Geometry check sheet. Reference: the model listing, model coordinates, mm. Face numbers are marked on the shaded views. Round coordinates to 2 decimals unless told otherwise and drop trailing zeros. Loops run counter-clockwise (first coordinate to the right, second up) from the corner with the lowest first, then second, coordinate; pieces in that order, holes last. Notation, with made-up numbers: (33.25, 70) -> (41.25, 70) arc R5 ccw to (41.25, 75) -> close; hole circle Ø10 at (69, 40). An arc over 180 degrees is marked (long way). Use a Markdown table: item, result. Add a question column.
Q1. Material ranges on L1, parallel to X at y = 41, z = 0; L2, parallel to X at y = 7, z = 0; L3, parallel to Y at x = -36.4, z = 0, recorded low to high.
Q2. Sectioned sample at C-C, the plane y = 36.5. Enter the section's corners in (x, z) (3 decimals), then the cut area to 3 significant figures.
Q3. Release check for a two-part mould opening along Z. For the marked faces 1, 2 and 3 record: released by +Z, released by -Z, zero draft, split by the parting line, or undercut.
Q4. Gauge pin test, flat ends, axial feed: P1, Ø12, axis at x = 10.5, z = -10, coming from the -Y side; P2, Ø6, axis at x = 21.5, z = 23.5, coming from the +Y side; P3, Ø8, axis at x = 9.5, z = -27.5, coming from the +Y side; P4, Ø24, axis at y = 20, z = 0, coming from the -X side. Record the tip position at first contact, or that the pin passes through.
Q5. Sectioned sample at B-B, the plane z = 0. Enter the section's corners in (x, y).
Q6. Sectioned sample at A-A, the plane x = 0. Enter the section's corners in (y, z), then the cut area to 3 significant figures.
Q7. Sectioned sample at D-D, the plane y = 20. Enter the section's corners in (x, z) (3 decimals), then the cut area to 3 significant figures.
```python
from build123d import *

# Parameters (mm, degrees)
SKETCH1_R           = 35.75
SKETCH1_R_2         = 34.75
BOSS_EXTRUDE1_DEPTH = 10
SKETCH2_R           = 36.8
SKETCH2_R_2         = 34.75
BOSS_EXTRUDE3_DEPTH = 2
SKETCH3_R           = 36.8
SKETCH3_R_2         = 35.8
BOSS_EXTRUDE4_DEPTH = 70
SKETCH4_W           = 1
SKETCH4_H           = 68.749981818
BOSS_EXTRUDE5_DEPTH = 50
SKETCH5_R           = 7.5
CUT_EXTRUDE1_DEPTH  = 10


with BuildPart() as part:
    # Sketch1 → Boss-Extrude1 (new body)
    with BuildSketch(Plane(origin=(0, 0, 0), x_dir=(1, 0, 0), z_dir=(0, 1, 0))):
        with Locations(Location((0, 0, 0), (0, 0, 270))):
            Circle(SKETCH1_R)
        with Locations(Location((0, 0, 0), (0, 0, 270))):
            Circle(SKETCH1_R_2, mode=Mode.SUBTRACT)
    extrude(amount=BOSS_EXTRUDE1_DEPTH)

    # Sketch2 → Boss-Extrude3 (add)
    with BuildSketch(Plane(origin=(0, 10, 0), x_dir=(1, 0, 0), z_dir=(0, 1, 0))):
        with Locations(Location((0, 0, 0), (0, 0, 270))):
            Circle(SKETCH2_R)
        with Locations(Location((0, 0, 0), (0, 0, 270))):
            Circle(SKETCH2_R_2, mode=Mode.SUBTRACT)
    extrude(amount=BOSS_EXTRUDE3_DEPTH)

    # Sketch3 → Boss-Extrude4 (add)
    with BuildSketch(Plane(origin=(0, 12, 0), x_dir=(1, 0, 0), z_dir=(0, 1, 0))):
        with Locations(Location((0, 0, 0), (0, 0, 270))):
            Circle(SKETCH3_R)
        with Locations(Location((0, 0, 0), (0, 0, 270))):
            Circle(SKETCH3_R_2, mode=Mode.SUBTRACT)
    extrude(amount=BOSS_EXTRUDE4_DEPTH)

    # Sketch4 → Boss-Extrude5 (add)
    with BuildSketch(Plane(origin=(0, 12, 0), x_dir=(1, 0, 0), z_dir=(0, 1, 0))):
        with Locations((10.5, 0)):
            Rectangle(SKETCH4_W, SKETCH4_H)
    extrude(amount=BOSS_EXTRUDE5_DEPTH)

    # Sketch5 → Cut-Extrude1 (cut)
    with BuildSketch(Plane.ZY.offset(36.8)):
        with Locations((0, 20)):
            Circle(SKETCH5_R)
    extrude(amount=-CUT_EXTRUDE1_DEPTH, mode=Mode.SUBTRACT)


solid = part.part
```
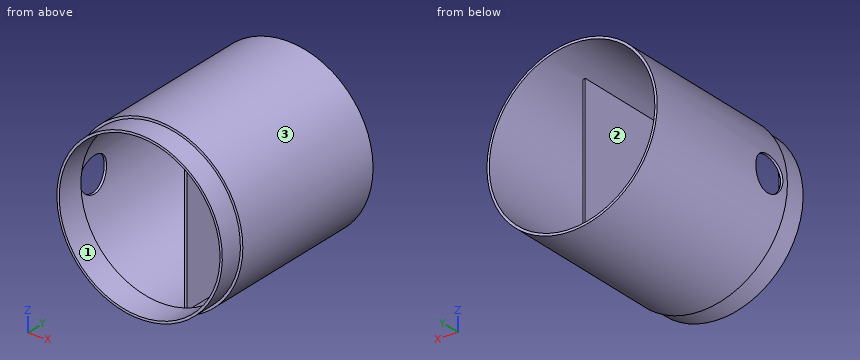
Values:
| question | item | result |
|---|---|---|
| 1 | L1 | -36.8 to -35.8, 10 to 11, 35.8 to 36.8 |
| 1 | L2 | -35.75 to -34.75, 34.75 to 35.75 |
| 1 | L3 | 10 to 12.5, 27.5 to 82 |
| 2 | outline | circle Ø73.6 at (0, 0); hole (10, -34.375) -> (10, 34.375) arc R35.8 ccw (long way) to start; hole (11, -34.068) arc R35.8 ccw to (11, 34.068) -> close |
| 2 | area | 297 mm^2 |
| 3 | face 1 | undercut |
| 3 | face 2 | undercut |
| 3 | face 3 | split by the parting line |
| 4 | P1 | y = 12 |
| 4 | P2 | y = 12 |
| 4 | P3 | y = 62 |
| 4 | P4 | x = -36.8 |
| 5 | outline | (-36.8, 10) -> (-35.75, 10) -> (-35.75, 0) -> (-34.75, 0) -> (-34.75, 12) -> (-35.8, 12) -> (-35.8, 12.5) -> (-36.8, 12.5) -> close; (-36.8, 27.5) -> (-35.8, 27.5) -> (-35.8, 82) -> (-36.8, 82) -> close; (10, 12) -> (11, 12) -> (11, 62) -> (10, 62) -> close; (34.75, 0) -> (35.75, 0) -> (35.75, 10) -> (36.8, 10) -> (36.8, 82) -> (35.8, 82) -> (35.8, 12) -> (34.75, 12) -> close |
| 6 | outline | (0, -35.75) -> (10, -35.75) -> (10, -36.8) -> (82, -36.8) -> (82, -35.8) -> (12, -35.8) -> (12, -34.75) -> (0, -34.75) -> close; (0, 34.75) -> (12, 34.75) -> (12, 35.8) -> (82, 35.8) -> (82, 36.8) -> (10, 36.8) -> (10, 35.75) -> (0, 35.75) -> close |
| 6 | area | 168 mm^2 |
| 7 | outline | (-36.028, -7.5) arc R36.8 ccw (long way) to (-36.028, 7.5) -> (-35.006, 7.5) arc R35.8 cw to (10, 34.375) -> (10, -34.375) arc R35.8 cw to (-35.006, -7.5) -> close; hole (11, -34.068) arc R35.8 ccw to (11, 34.068) -> close |
| 7 | area | 281 mm^2 |
